from build123d import *

# Parameters (mm, degrees)
F0_W      = 22.225
F0_H      = 69.85
F1_DEPTH  = 57.15
F2_W      = 22.225
F2_H      = 12.7
F3_DEPTH  = 1.5875
F4_R      = 6.35
F5_W      = 3.175
F5_H      = 6.35
F6_DEPTH  = 25.4
F7_R      = 1.58749
F8_W      = 44.45
F8_H      = 31.75
F10_DEPTH = 12.7
F9_W      = 44.45
F9_H      = 31.75
F11_DEPTH = 12.7
F12_R     = 5.715
F13_R     = 1.5875


# Not quite as in the source:
# - a fillet or chamfer is up to 0.001 mm smaller than in the source, because OpenCascade refuses the exact size


with BuildPart() as f1:
    # F0 (on Top) → F1 (new body)
    with BuildSketch(Plane.XY):
        Rectangle(F0_W, F0_H)
    extrude(amount=F1_DEPTH)

    # F2 (on face) → F3 (join)
    with BuildSketch(Plane(origin=(0, 0, 0), x_dir=(1, 0, 0), z_dir=(0, 0, -1))):
        with Locations((0, 41.275)):
            Rectangle(F2_W, F2_H)
        with Locations((0, -41.275)):
            Rectangle(F2_W, F2_H)
    extrude(amount=-F3_DEPTH)

    # F4
    f4_edges = [f1.edges().sort_by_distance(p)[0] for p in [
        (-11.1125, -47.625, 0.79375),
        (11.1125, -47.625, 0.79375),
        (-11.1125, 47.625, 0.79375),
        (11.1125, 47.625, 0.79375),
    ]]
    fillet(f4_edges, radius=F4_R)

    # F5 (on face) → F6 (cut)
    with BuildSketch(Plane.XY.offset(1.5875)):
        with Locations((0, 41.275)):
            Rectangle(F5_W, F5_H)
        with Locations((0, -41.275)):
            Rectangle(F5_W, F5_H)
    extrude(amount=-F6_DEPTH, mode=Mode.SUBTRACT)

    # F7 (radius 1.5875 in the source; OpenCascade refuses exactly that, so slightly less here)
    f7_edges = [f1.edges().sort_by_distance(p)[0] for p in [
        (1.5875, 44.45, 0.79375),
        (-1.5875, 44.45, 0.79375),
        (-1.5875, 38.1, 0.79375),
        (1.5875, 38.1, 0.79375),
        (1.5875, -38.1, 0.79375),
        (-1.5875, -38.1, 0.79375),
        (-1.5875, -44.45, 0.79375),
        (1.5875, -44.45, 0.79375),
    ]]
    fillet(f7_edges, radius=F7_R)

    # F8 (on face) → F10 (join)
    with BuildSketch(Plane.YZ.offset(11.1125)):
        with Locations((0, 28.575)):
            Rectangle(F8_W, F8_H)
    extrude(amount=F10_DEPTH)

    # F9 (on face) → F11 (join)
    with BuildSketch(Plane(origin=(-11.1125, 0, 0), x_dir=(0, -1, 0), z_dir=(-1, 0, 0))):
        with Locations((0, 28.575)):
            Rectangle(F9_W, F9_H)
    extrude(amount=F11_DEPTH)

    # F12
    f12_edges = [f1.edges().sort_by_distance(p)[0] for p in [
        (23.8125, -22.225, 28.575),
        (23.8125, 22.225, 28.575),
        (-23.8125, -22.225, 28.575),
        (-23.8125, 22.225, 28.575),
    ]]
    fillet(f12_edges, radius=F12_R)

    # F13
    f13_edges = [f1.edges().sort_by_distance(p)[0] for p in [
        (11.1125, -34.925, 29.36875),
        (11.1125, 0, 57.15),
        (11.1125, 34.925, 29.36875),
        (0, -34.925, 57.15),
        (0, 34.925, 57.15),
        (-11.1125, -34.925, 29.36875),
        (-11.1125, 0, 57.15),
        (-11.1125, 34.925, 29.36875),
    ]]
    fillet(f13_edges, radius=F13_R)


solid = f1.part
Could you check a few things on this model? Use its own coordinates, in mm. A direction names the side the tool comes from. Round coordinates to 2 decimals unless told otherwise and drop trailing zeros. Order: outer loops, then holes, each group sorted by start corner. A loop starts at its lowest first (then second) coordinate and runs counter-clockwise, first axis right, second up. Notation, with made-up numbers: M 18,24 L 24,24 A13 ccw 24,49 Z; hole C 32.25,44.25 d2. An arc over 180 degrees is marked long. One line per item, written item: value.
(1) I need wall thicknesses on line 1 along Y through (x, z) = (6.5, 46) (3 decimals); line 2 along X through (y, z) = (6, 10.5); line 3 along Y through (x, z) = (-11.5, 22) (3 decimals). Which ranges of each line are inside material? Lowest first, please. Write a range as from..to.
Ans:
line 1: y = -34.925..34.925
line 2: x = -11.11..11.11
line 3: y = -22.225..22.225
(2) I'm going to push flat-ended pins straight in: P1, Ø1.5, axis at x = 11, z = 44, coming from the +Y side; P2, Ø10, axis at x = 19, y = 3.5, coming from the +Z side; P3, Ø1.5, axis at x = 13, y = -12.5, coming from the -Z side. Where does each tip first touch, or does it pass through?
Ans:
P1: stops at y = 34.75
P2: stops at z = 44.45
P3: stops at z = 12.7
(3) Which directions (+Z, -Z, +X, -X, +Y, -Y) give clear straight access to the entire face, cutting with the end or side of a thin tool? Please do faces 1 (the flat face through (17, 0, 44.45)), 2 (the flat face through (-17, 0, 12.7)), 3 (the flat face through (0, -34.925, 28)), 4 (the flat face through (15, 22.225, 28)), 5 (the flat face through (-17, 0, 44.45)).
Ans:
face 1: +Z, +X, +Y, -Y
face 2: -Z, -X, +Y, -Y
face 3: +Z, +X, -X, -Y
face 4: +Z, -Z, +X, +Y
face 5: +Z, -X, +Y, -Y
(4) Imagine slicing it at B-B (z = 51.5). Write out the boundary of the cut face in (x, y) (1 decimal), and give its area (3 significant figures).
Ans:
outline: M -11.1,-33.3 A1.6 ccw -9.5,-34.9 L 9.5,-34.9 A1.6 ccw 11.1,-33.3 L 11.1,33.3 A1.6 ccw 9.5,34.9 L -9.5,34.9 A1.6 ccw -11.1,33.3 Z
area: 1,550 mm^2
